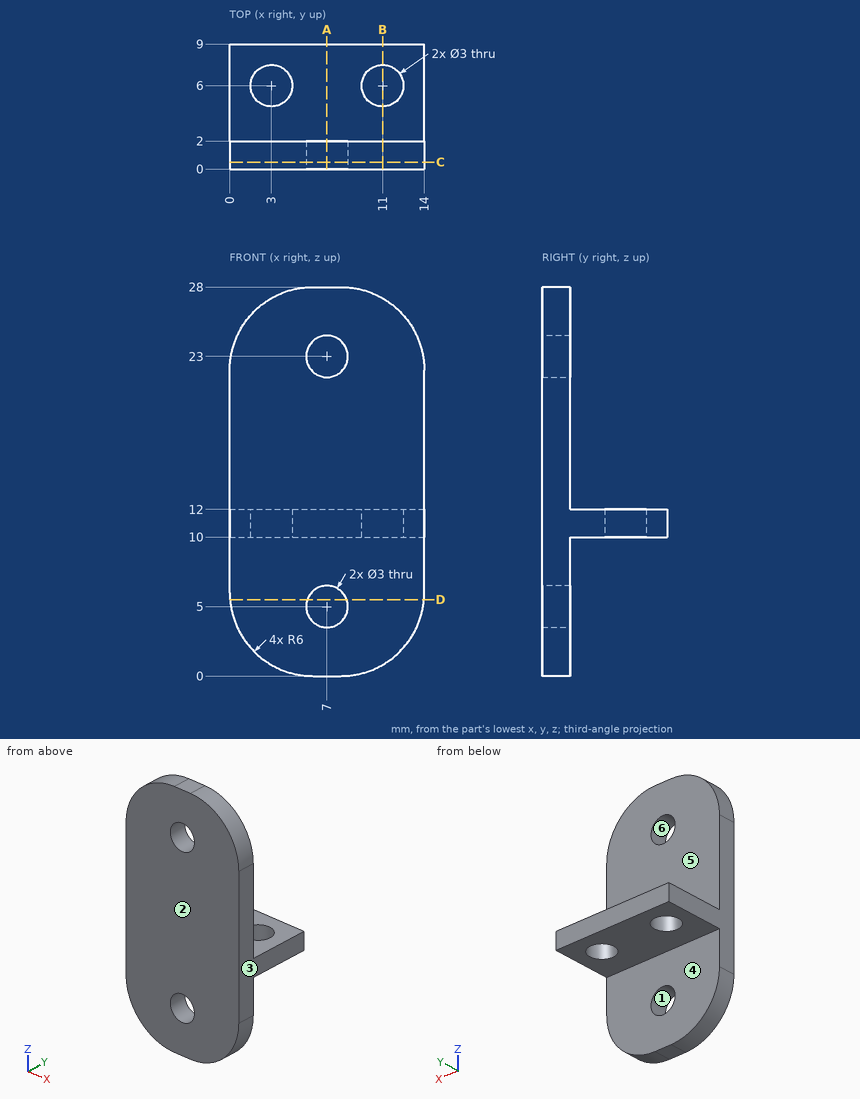
Study the drawing (mm; zero at the part's minimum x, y, z) and answer. A direction names the side the tool comes from. Give positions to 0.01 mm unless a question says otherwise; leave off trailing zeros. Order: outer loops, then holes, each group sorted by start corner. A loop starts at its lowest first (then second) coordinate and runs counter-clockwise, first axis right, second up. Notation, with made-up numbers: (23, 8) - (29, 8) arc R21 cw to (29, 44) - close; hole circle Ø6 at (66.25, 76.5). An arc over 180 degrees is marked (long way). Use one line per item in the form item = value. Start each with the question number.
(1) Consider line 1 (Y direction, x = 11, z = 10.85); line 2 (Y direction, x = 1, z = 22); line 3 (Z direction, x = 7.75, y = 4). Determine where each line is inside the solid, lowest interval first. Write a range as from..to.
(2) A cutting plane is placed at B-B, the plane x = 11. Write down the section's boundary in (y, z).
(3) A cutting plane is placed at A-A, the plane x = 7. Write down the section's boundary in (y, z), then the cut area to 3 significant figures.
(4) Flat-ended cylindrical pins translate along their axes: pin 1 Ø4 at (x, y) = (3, 6) entering from +Z; pin 2 Ø5 at (x, z) = (8, 6) entering from +Y; pin 3 Ø6 at (x, z) = (12, 3) entering from -Y; pin 4 Ø2 at (x, y) = (6, 7) entering from -Z. Find the tip coordinate at first contact, or state that the pin passes through.
(5) For the marked faces 4, 5 and 6, determine the directions among +Z, -Z, +X, -X, +Y, -Y from which every point of the face is accessible in a straight line to the end or side of a thin tool.
(6) A cutting plane is placed at C-C, the plane y = 0.5. Write down the section's boundary in (x, z).
(7) A cutting plane is placed at D-D, the plane z = 5.5. Write down the section's boundary in (x, y), then the cut area to 3 significant figures.
(8) The mould has two halves that part along X. Classify the marked faces 1, 2 and 3: released by +X, released by -X, zero draft, split by the parting line, or undercut.
Ans:
q1.line_1 = 0..4.5, 7.5..9
q1.line_2 = 0..2
q1.line_3 = 10..12
q2.outline = (0, 0.8) - (2, 0.8) - (2, 10) - (4.5, 10) - (4.5, 12) - (2, 12) - (2, 27.2) - (0, 27.2) - close; (7.5, 10) - (9, 10) - (9, 12) - (7.5, 12) - close
q3.outline = (0, 0) - (2, 0) - (2, 3.5) - (0, 3.5) - close; (0, 6.5) - (2, 6.5) - (2, 10) - (9, 10) - (9, 12) - (2, 12) - (2, 21.5) - (0, 21.5) - close; (0, 24.5) - (2, 24.5) - (2, 28) - (0, 28) - close
q3.area = 58.0 mm^2
q4.pin_1 = 12
q4.pin_2 = 2
q4.pin_3 = 0
q4.pin_4 = 10
q5.face_4 = -Z, +X, -X, +Y
q5.face_5 = +Z, +X, -X, +Y
q5.face_6 = +Y, -Y
q6.outline = (0, 6) arc R6 ccw to (6, 0) - (8, 0) arc R6 ccw to (14, 6) - (14, 22) arc R6 ccw to (8, 28) - (6, 28) arc R6 ccw to (0, 22) - close; hole circle Ø3 at (7, 5); hole circle Ø3 at (7, 23)
q7.outline = (0.02, 0) - (5.59, 0) - (5.59, 2) - (0.02, 2) - close; (8.41, 0) - (13.98, 0) - (13.98, 2) - (8.41, 2) - close
q7.area = 22.3 mm^2
q8.face_1 = undercut
q8.face_2 = zero draft
q8.face_3 = released by +X
